Work out the finished part from the listing and answer in its coordinate system (mm). A direction names the side the tool comes from. Round coordinates to 2 decimals unless told otherwise and drop trailing zeros. Write each loop counter-clockwise with the first axis right and the second up, starting at its lowest first coordinate (ties: lowest second). Pieces come first, ordered by that corner, then holes. Notation, with made-up numbers: M -39.75,59.25 L 9.25,59.25 A20 cw 9.25,81.25 Z; hole C -10.5,87.5 d6. An arc over 180 degrees is marked long. One line per item, written item: value. Start each with the question number.
Q1. Consider probe 1 along Y at (x, z) = (20, 55.5); probe 2 along Y at (x, z) = (-27.6, 0). Determine where each line is inside the solid, lowest interval first.
Q2. Find section A-A (x = 4.5). Write down the section's boundary in (y, z).
Q3. The mould has two halves that part along Y. Classify faces 4 (the flat face through (0, -30, 1)), 5 (the flat face through (-30, -7, 1)), 6 (the flat face through (26, 0, 1)), 7 (the flat face through (0, 26, 1)): released by +Y, released by -Y, zero draft, split by the parting line, or undercut.
Q4. Given pin 1 Ø12 at (x, y) = (-13.5, -16) entering from +Z, flat-ended and moving along its own axis, determine where the tip first touches the part or whether it passes through.
Q5. A tool of negligible diameter and unlimited length cuts with its end or side. For faces 1 (the flat face through (-27, 0, 75)), 2 (the flat face through (-26, -6, 1)), 3 (the cylindrical face through (-28.03, -4.88, -1.08)), from which of +Z, -Z, +X, -X, +Y, -Y can it reach the whole face along a straight path? Write none if from no direction.
Q6. Find section B-B (y = 0). Write down the section's boundary in (x, z).
Q7. Find section D-D (z = -19). Write down the section's boundary in (x, y), and give its area (3 significant figures).
from build123d import *

# Parameters (mm, degrees)
SZKIC1_W                    = 60
SZKIC1_H                    = 60
SZKIC1_W_2                  = 52
SZKIC1_H_2                  = 52
DODANIE_WYCI_GNI_CIE1_DEPTH = 75
SZKIC28_R                   = 5
WYTNIJ_WYCI_GNI_CIE1_DEPTH  = 25


with BuildPart() as part:
    # Szkic1 → Dodanie-wyciągnięcie1 (new body, symmetric)
    with BuildSketch(Plane.XY):
        Rectangle(SZKIC1_W, SZKIC1_H)
        Rectangle(SZKIC1_W_2, SZKIC1_H_2, mode=Mode.SUBTRACT)
    extrude(amount=DODANIE_WYCI_GNI_CIE1_DEPTH, both=True)

    # Szkic28 → Wytnij-wyciągnięcie1 (cut)
    with BuildSketch(Plane.ZY.offset(30)):
        Circle(SZKIC28_R)
    extrude(amount=-WYTNIJ_WYCI_GNI_CIE1_DEPTH, mode=Mode.SUBTRACT)


solid = part.part
The answers:
1. probe 1: -30 to -26, 26 to 30
1. probe 2: -30 to -5, 5 to 30
2. outline: M -30,-75 L -26,-75 L -26,75 L -30,75 Z; M 26,-75 L 30,-75 L 30,75 L 26,75 Z
3. face 4: released by -Y
3. face 5: zero draft
3. face 6: undercut
3. face 7: undercut
4. pin 1: through
5. face 1: +Z, +X, -X, +Y, -Y
5. face 2: +Z, -Z
5. face 3: -X
6. outline: M -30,-75 L -26,-75 L -26,-5 L -30,-5 Z; M -30,5 L -26,5 L -26,75 L -30,75 Z; M 26,-75 L 30,-75 L 30,75 L 26,75 Z
7. outline: M -30,-30 L 30,-30 L 30,30 L -30,30 Z; hole M -26,-26 L 26,-26 L 26,26 L -26,26 Z
7. area: 896 mm2
